Geometry check sheet. Reference: the model listing, model coordinates, mm. A direction names the side the tool comes from. Coordinates: 2 decimals unless noted, no trailing zeros. Write each loop counter-clockwise with the first axis right and the second up, starting at its lowest first coordinate (ties: lowest second). Pieces come first, ordered by that corner, then holes.
from build123d import *

# Parameters (mm, degrees)
SKETCH1_W           = 12
SKETCH1_H           = 12
BOSS_EXTRUDE1_DEPTH = 3.25
CHAMFER1_SIZE       = 1
SKETCH2_W           = 5
SKETCH2_H           = 5
BOSS_EXTRUDE2_DEPTH = 3
SKETCH3_R           = 6.5
BOSS_EXTRUDE3_DEPTH = 5.5
CUT_EXTRUDE1_START  = -4.2
SKETCH4_R           = 6.5
SKETCH4_R_2         = 5.725
CUT_EXTRUDE1_DEPTH  = 4.2
FILLET1_R           = 0.5


with BuildPart() as part:
    # Sketch1 → Boss-Extrude1 (new body)
    with BuildSketch(Plane(origin=(0, 0, 0), x_dir=(1, 0, 0), z_dir=(0, 1, 0))):
        Rectangle(SKETCH1_W, SKETCH1_H)
    extrude(amount=BOSS_EXTRUDE1_DEPTH)

    # Chamfer1
    chamfer1_edges = [part.edges().sort_by_distance(p)[0] for p in [
        (-6, 1.625, -6),
        (6, 1.625, -6),
        (6, 1.625, 6),
        (-6, 1.625, 6),
    ]]
    chamfer(chamfer1_edges, length=CHAMFER1_SIZE)

    # Sketch2 → Boss-Extrude2 (add)
    with BuildSketch(Plane(origin=(0, 3.25, 0), x_dir=(1, 0, 0), z_dir=(0, 1, 0))):
        Rectangle(SKETCH2_W, SKETCH2_H)
    extrude(amount=BOSS_EXTRUDE2_DEPTH)

    # Sketch3 → Boss-Extrude3 (add)
    with BuildSketch(Plane(origin=(0, 6.25, 0), x_dir=(1, 0, 0), z_dir=(0, 1, 0))):
        with Locations(Location((0, 0, 0), (0, 0, 270))):
            Circle(SKETCH3_R)
    extrude(amount=BOSS_EXTRUDE3_DEPTH)

    # Sketch4 → Cut-Extrude1 (cut)
    with BuildSketch(Plane(origin=(0, 11.75, 0), x_dir=(1, 0, 0), z_dir=(0, 1, 0)).offset(CUT_EXTRUDE1_START)):
        with Locations(Location((0, 0, 0), (0, 0, 270))):
            Circle(SKETCH4_R)
        with Locations(Location((0, 0, 0), (0, 0, 270))):
            Circle(SKETCH4_R_2, mode=Mode.SUBTRACT)
    extrude(amount=CUT_EXTRUDE1_DEPTH, mode=Mode.SUBTRACT)

    # Fillet1
    fillet1_edges = [part.edges().sort_by_distance(p)[0] for p in [
        (0, 11.75, -5.725),
    ]]
    fillet(fillet1_edges, radius=FILLET1_R)


solid = part.part
1. Sectioned sample at D-D, the plane y = 7.25. Record the boundary of the cut face in (x, z).
Computed values:
outline: circle Ø13 at (0, 0)
2. Sectioned sample at B-B, the plane x = 0. Record the boundary of the cut face in (y, z) (3 decimals), and give its area (3 significant figures).
Computed values:
outline: (0, -6) - (3.25, -6) - (3.25, -2.5) - (6.25, -2.5) - (6.25, -6.5) - (7.55, -6.5) - (7.55, -5.725) - (11.25, -5.725) arc R0.5 ccw to (11.75, -5.225) - (11.75, 5.225) arc R0.5 ccw to (11.25, 5.725) - (7.55, 5.725) - (7.55, 6.5) - (6.25, 6.5) - (6.25, 2.5) - (3.25, 2.5) - (3.25, 6) - (0, 6) - close
area: 119 mm2
3. Sectioned sample at C-C, the plane z = 0. Record the boundary of the cut face in (x, y) (3 decimals), and give its area (3 significant figures).
Computed values:
outline: (-6.5, 6.25) - (-2.5, 6.25) - (-2.5, 3.25) - (-6, 3.25) - (-6, 0) - (6, 0) - (6, 3.25) - (2.5, 3.25) - (2.5, 6.25) - (6.5, 6.25) - (6.5, 7.55) - (5.725, 7.55) - (5.725, 11.25) arc R0.5 ccw to (5.225, 11.75) - (-5.225, 11.75) arc R0.5 ccw to (-5.725, 11.25) - (-5.725, 7.55) - (-6.5, 7.55) - close
area: 119 mm2
4. Access from +Z, -Z, +X, -X, +Y, -Y to the whole of each face (thin tool, end or side, straight path). Record for faces 4 (the flat face through (2.5, 5, 0)), 5 (the flat face through (0, 5, 2.5)), 6 (the flat face through (0, 6.25, 3)), 7 (the flat face through (6, 2, 0)).
Computed values:
face 4: +Z, -Z, +X
face 5: +Z, +X, -X
face 6: none
face 7: +Z, -Z, +X, -Y
5. Sectioned sample at A-A, the plane y = 2. Record the boundary of the cut face in (x, z), and give its area (3 significant figures).
Computed values:
outline: (-6, -5) - (-5, -6) - (5, -6) - (6, -5) - (6, 5) - (5, 6) - (-5, 6) - (-6, 5) - close
area: 142 mm2
6. Gauge pin test, flat ends, axial feed: pin 1 Ø2.5 at (x, y) = (0, 4) entering from -Z; pin 2 Ø5 at (x, y) = (-2.5, 6) entering from +Z; pin 3 Ø1.6 at (x, y) = (-0.5, 1) entering from +Z; pin 4 Ø2.5 at (y, z) = (2.5, 1) entering from -X. Record the tip position at first contact, or that the pin passes through.
Computed values:
pin 1: stops at z = -6
pin 2: stops at z = 6.5
pin 3: stops at z = 6
pin 4: stops at x = -6
7. Thickness scan on line 1 along Y through (x, z) = (4, 4.5); line 2 along Y through (x, z) = (3.25, 3); line 3 along Z through (x, y) = (3, 0.5). Record the ranges inside material, lowest first.
Computed values:
line 1: y = 0 to 3.25, 6.25 to 7.55
line 2: y = 0 to 3.25, 6.25 to 11.75
line 3: z = -6 to 6
8. Draft check along Y on faces 1 (the flat face through (0, 5, -2.5)), 2 (the flat face through (-5.5, 1.6, -5.5)), 3 (the flat face through (0, 11.75, 0)). Enter one of: released by +Y, released by -Y, zero draft, split by the parting line, or undercut.
Computed values:
face 1: undercut
face 2: zero draft
face 3: released by +Y
